Check sheet for the modelled part. Datum: model origin and axes. Units: mm. A direction names the side the tool comes from. Round coordinates to 2 decimals unless told otherwise and drop trailing zeros. Order: outer loops, then holes, each group sorted by start corner. A loop starts at its lowest first (then second) coordinate and runs counter-clockwise, first axis right, second up.
(1) Sectioned sample at C-C, the plane x = 48. Enter the section's corners in (y, z), and give its area (3 significant figures).
(2) Sectioned sample at B-B, the plane x = 9. Enter the section's corners in (y, z), and give its area (3 significant figures).
(3) Sectioned sample at A-A, the plane z = -4.65. Enter the section's corners in (x, y).
(4) Depth check by flat-ended pin: pin 1 (1.9 mm diameter, centred on y = 15.5, z = -35.65, fed in from -X); pin 2 (5 mm diameter, centred on y = -15.5, z = -35.65, fed in from -X); pin 3 (12.5 mm diameter, centred on x = 11, y = 7.5, fed in from -Z); pin 4 (18.5 mm diameter, centred on y = 0, z = -20.15, fed in from +X). Enter the tip coordinate at first touch or a pass-through.
(5) Thickness scan on probe 1 along Y at (x, z) = (73.5, -4.65); probe 2 along Y at (x, z) = (72, -20); probe 3 along Y at (x, z) = (-4, 7). Record the ranges inside material, lowest first.
(6) Mould release check, pull along X, two halves, no side actions. Record for faces 4 (the cylindrical face through (-21, 0, 4)), 5 (the cylindrical face through (-4.71, 9.38, 5.42)), 6 (the cylindrical face through (74.93, -14.42, -36.83)): released by +X, released by -X, zero draft, split by the parting line, or undercut.
(7) Sectioned sample at D-D, the plane z = 5. Enter the section's corners in (x, y).
(8) Tool access check on faces 1 (the cylindrical face through (11.923, 3.755, 0.493)), 2 (the flat face through (3, 0, 0)), 3 (the cylindrical face through (71.5, 7.8, -28.6)). Record the directions out of +Z, -Z, +X, -X, +Y, -Y that give a thin tool (end or side, any length) a straight path to the whole face; none if there is none.
```python
from build123d import *

# Parameters (mm, degrees)
SKETCH_1_R          = 12.5
SKETCH_1_R_2        = 1.6
EXTRUDE_1_DEPTH     = 11
SKETCH_2_R          = 12.5
EXTRUDE_2_DEPTH     = 10
SKETCH_3_W          = 52.3
SKETCH_3_H          = 42
EXTRUDE_3_DEPTH     = 10
SKETCH_6_R          = 2.6
CUT_EXTRUDE_1_DEPTH = 53.3
SKETCH_8_R          = 1.6
SKETCH_8_R_2        = 2.6
CUT_EXTRUDE_3_DEPTH = 11
SKETCH_9_R          = 11.5
CUT_EXTRUDE_4_DEPTH = 3
CHAMFER_1_SIZE      = 5
CHAMFER_2_SIZE      = 4.2


with BuildPart() as part:
    # 草图1 → 凸台-拉伸1 (new body)
    with BuildSketch(Plane.XY):
        Circle(SKETCH_1_R)
        with Locations((9, 0)):
            Circle(SKETCH_1_R_2, mode=Mode.SUBTRACT)
        with Locations((-4.5, -7.794228634)):
            Circle(SKETCH_1_R_2, mode=Mode.SUBTRACT)
        with Locations((-4.5, 7.794228634)):
            Circle(SKETCH_1_R_2, mode=Mode.SUBTRACT)
    extrude(amount=EXTRUDE_1_DEPTH)

    # 草图2 → 凸台-拉伸2 (add)
    with BuildSketch(Plane.XY.offset(11)):
        with BuildLine():
            Line((0, 21), (70, 21))
            Line((70, 21), (70, -21))
            Line((70, -21), (0, -21))
            ThreePointArc((0, -21), (-21, 0), (0, 21))
        make_face()
        Circle(SKETCH_2_R, mode=Mode.SUBTRACT)
    extrude(amount=-EXTRUDE_2_DEPTH)

    # 草图3 → 凸台-拉伸3 (add)
    with BuildSketch(Plane(origin=(70, 0, 0), x_dir=(0, 0, -1), z_dir=(1, 0, 0))):
        with Locations((15.15, 0)):
            Rectangle(SKETCH_3_W, SKETCH_3_H)
    extrude(amount=EXTRUDE_3_DEPTH)

    # 草图6 → 切除-拉伸1 (cut, through all)
    with BuildSketch(Plane(origin=(0, 0, -41.3), x_dir=(-1, 0, 0), z_dir=(0, 0, -1))):
        Circle(SKETCH_6_R)
    extrude(amount=-CUT_EXTRUDE_1_DEPTH, mode=Mode.SUBTRACT)

    # 草图8 → 切除-拉伸3 (cut, through all)
    with BuildSketch(Plane.ZY.offset(-70)):
        with Locations((-35.65, 15.5)):
            Circle(SKETCH_8_R)
        with Locations((-4.65, 15.5)):
            Circle(SKETCH_8_R)
        with Locations((-4.65, -15.5)):
            Circle(SKETCH_8_R)
        with Locations((-35.65, -15.5)):
            Circle(SKETCH_8_R)
        with Locations((-20.15, 0)):
            Circle(SKETCH_8_R_2)
    extrude(amount=-CUT_EXTRUDE_3_DEPTH, mode=Mode.SUBTRACT)

    # 草图9 → 切除-拉伸4 (cut)
    with BuildSketch(Plane.ZY.offset(-70)):
        with Locations((-20.15, 0)):
            Circle(SKETCH_9_R)
    extrude(amount=-CUT_EXTRUDE_4_DEPTH, mode=Mode.SUBTRACT)

    # 倒角1
    chamfer_1_edges = [part.edges().sort_by_distance(p)[0] for p in [
        (-21, 0, 11),
        (40, -21, 11),
        (40, 21, 11),
    ]]
    chamfer(chamfer_1_edges, length=CHAMFER_1_SIZE)

    # 倒角2
    chamfer_2_edges = [part.edges().sort_by_distance(p)[0] for p in [
        (75, -21, -41.3),
        (75, 21, -41.3),
    ]]
    chamfer(chamfer_2_edges, length=CHAMFER_2_SIZE)


solid = part.part
```
Derived:
1. outline: (-21, 1) - (21, 1) - (21, 6) - (16, 11) - (-16, 11) - (-21, 6) - close
1. area: 395 mm2
2. outline: (-21, 1) - (-8.67, 1) - (-8.67, 0) - (-1.6, 0) - (-1.6, 11) - (-16, 11) - (-21, 6) - close; (1.6, 0) - (8.67, 0) - (8.67, 1) - (21, 1) - (21, 6) - (16, 11) - (1.6, 11) - close
2. area: 377 mm2
3. outline: (70, -21) - (80, -21) - (80, -17.1) - (70, -17.1) - close; (70, -13.9) - (80, -13.9) - (80, 13.9) - (70, 13.9) - close; (70, 17.1) - (80, 17.1) - (80, 21) - (70, 21) - close
4. pin 1: passes through
4. pin 2: stops at x = 70
4. pin 3: stops at z = 0
4. pin 4: stops at x = 80
5. probe 1: y = -21 to -17.1, -13.9 to 13.9, 17.1 to 21
5. probe 2: y = -21 to -11.5, 11.5 to 21
5. probe 3: y = -19.6 to -9.31, -6.27 to 6.27, 9.31 to 19.6
6. face 4: released by -X
6. face 5: undercut
6. face 6: zero draft
7. outline: (0, -21) - (80, -21) - (80, 21) - (0, 21) arc R21 ccw to start; hole circle Ø3.2 at (-4.5, -7.79); hole circle Ø3.2 at (-4.5, 7.79); hole circle Ø5.2 at (0, 0); hole circle Ø3.2 at (9, 0)
8. face 1: -Z
8. face 2: -Z, -X, +Y, -Y
8. face 3: -X
